from build123d import *

# Parameters (mm, degrees)
CROQUIS1_R              = 4.25
CROQUIS1_R_2            = 2
SALIENTE_EXTRUIR1_DEPTH = 14.2
CROQUIS2_W              = 12
CROQUIS2_H              = 162.31128511
CORTAR_EXTRUIR1_DEPTH   = 4
CROQUIS3_R              = 6.5
CORTAR_EXTRUIR2_DEPTH   = 8


with BuildPart() as part:
    # Croquis1 → Saliente-Extruir1 (new body)
    with BuildSketch(Plane.XY):
        with BuildLine():
            Line((69, -75), (56, -75))
            Line((56, -75), (56, -63))
            ThreePointArc((56, -63), (50, -57), (44, -63))
            Line((44, -63), (44, -75))
            Line((44, -75), (-44, -75))
            Line((-44, -75), (-44, -63))
            ThreePointArc((-44, -63), (-50, -57), (-56, -63))
            Line((-56, -63), (-56, -75))
            Line((-56, -75), (-69, -75))
            Line((-69, -75), (-69, 75))
            Line((-69, 75), (-56, 75))
            Line((-56, 75), (-56, 63))
            ThreePointArc((-56, 63), (-50, 57), (-44, 63))
            Line((-44, 63), (-44, 75))
            Line((-44, 75), (44, 75))
            Line((44, 75), (44, 63))
            ThreePointArc((44, 63), (50, 57), (56, 63))
            Line((56, 63), (56, 75))
            Line((56, 75), (69, 75))
            Line((69, 75), (69, -75))
        make_face()
        with Locations((-32.5, 40)):
            Circle(CROQUIS1_R, mode=Mode.SUBTRACT)
        with Locations((-32.5, 0)):
            Circle(CROQUIS1_R, mode=Mode.SUBTRACT)
        with Locations((-32.5, -40)):
            Circle(CROQUIS1_R, mode=Mode.SUBTRACT)
        with Locations((32.5, 40)):
            Circle(CROQUIS1_R, mode=Mode.SUBTRACT)
        with Locations((32.5, 0)):
            Circle(CROQUIS1_R, mode=Mode.SUBTRACT)
        with Locations((32.5, -40)):
            Circle(CROQUIS1_R, mode=Mode.SUBTRACT)
        with Locations((0, 65)):
            Circle(CROQUIS1_R_2, mode=Mode.SUBTRACT)
        Circle(CROQUIS1_R_2, mode=Mode.SUBTRACT)
        with Locations((0, -65)):
            Circle(CROQUIS1_R_2, mode=Mode.SUBTRACT)
    extrude(amount=SALIENTE_EXTRUIR1_DEPTH)

    # Croquis2 → Cortar-Extruir1 (cut)
    with BuildSketch(Plane.XY.offset(14.2)):
        with Locations((0, -0.838384737)):
            Rectangle(CROQUIS2_W, CROQUIS2_H)
    extrude(amount=-CORTAR_EXTRUIR1_DEPTH, mode=Mode.SUBTRACT)

    # Croquis3 → Cortar-Extruir2 (cut)
    with BuildSketch(Plane.XY.offset(14.2)):
        with Locations((-32.5, 40)):
            Circle(CROQUIS3_R)
        with Locations((-32.5, 0)):
            Circle(CROQUIS3_R)
        with Locations((-32.5, -40)):
            Circle(CROQUIS3_R)
        with Locations((32.5, 40)):
            Circle(CROQUIS3_R)
        with Locations((32.5, 0)):
            Circle(CROQUIS3_R)
        with Locations((32.5, -40)):
            Circle(CROQUIS3_R)
    extrude(amount=-CORTAR_EXTRUIR2_DEPTH, mode=Mode.SUBTRACT)


solid = part.part
Part model, mm, in its own coordinate system. A direction names the side the tool comes from. Round coordinates to 2 decimals unless told otherwise and drop trailing zeros. Order: outer loops, then holes, each group sorted by start corner. A loop starts at its lowest first (then second) coordinate and runs counter-clockwise, first axis right, second up. Notation, with made-up numbers: (-20.5, 88) -> (-7.5, 88) arc R6 cw to (-7.5, 98) -> close; hole circle Ø1 at (81.25, -5). An arc over 180 degrees is marked (long way). Put each result on its own line as item: value.
Q1. Pull direction Y, two halves, no side cores. Call faces 5 (the face through (56, -69, 7)), 6 (the face through (1, -75, 7)), 7 (the face through (33.9, -4.2, 6.2)), 8 (the face through (-39, 0, 10)): pulls with the +Y half, pulls with the -Y half, needs draft (parallel to the pull), parting line crosses it, or undercut.
From the geometry:
face 5: needs draft
face 6: pulls with the -Y half
face 7: undercut
face 8: undercut
Q2. Band-saw the part on C-C (y = -40). Give the cut face in (x, z), and give its area (3 significant figures).
From the geometry:
outline: (-69, 0) -> (-36.75, 0) -> (-36.75, 6.2) -> (-39, 6.2) -> (-39, 14.2) -> (-69, 14.2) -> close; (-28.25, 0) -> (28.25, 0) -> (28.25, 6.2) -> (26, 6.2) -> (26, 14.2) -> (6, 14.2) -> (6, 10.2) -> (-6, 10.2) -> (-6, 14.2) -> (-26, 14.2) -> (-26, 6.2) -> (-28.25, 6.2) -> close; (36.75, 0) -> (69, 0) -> (69, 14.2) -> (39, 14.2) -> (39, 6.2) -> (36.75, 6.2) -> close
area: 1,600 mm2
Q3. Wall check: line 1 (Y direction, x = -32.5, z = 11.25); line 2 (X direction, y = 69.5, z = 12); line 3 (X direction, y = 0, z = 3.25). Give the ranges that are in metal, low to high. Write a range as [from, to].
From the geometry:
line 1: y = [-75, -46.5], [-33.5, -6.5], [6.5, 33.5], [46.5, 75]
line 2: x = [-69, -56], [-44, -6], [6, 44], [56, 69]
line 3: x = [-69, -36.75], [-28.25, -2], [2, 28.25], [36.75, 69]
Q4. Tool access for faces 1 (the face through (3, 1, 10.2)), 2 (the face through (56, 69, 7)), 3 (the face through (31.654, -33.555, 10.256)), 4 (the face through (44, -69, 7)): list every direction of +Z, -Z, +X, -X, +Y, -Y with a clear straight run to the whole face (end or side of a thin tool).
From the geometry:
face 1: +Z, +Y, -Y
face 2: +Z, -Z, +Y
face 3: +Z
face 4: +Z, -Z, -Y
Q5. Pin check, flat tips, straight feed: pin 1 Ø5 at (x, y) = (-13, 32.5) entering from -Z; pin 2 Ø11 at (x, y) = (-32.5, 0) entering from +Z; pin 3 Ø4 at (x, z) = (48, 8) entering from -Y. Stop position of each tip, or through.
From the geometry:
pin 1: stops at z = 0
pin 2: stops at z = 6.2
pin 3: stops at y = -58.53
Q6. Band-saw the part on D-D (z = 3). State how many separate pieces and enclosed holes the cut face has, and give its area (3 significant figures).
From the geometry:
separate pieces: 1
enclosed holes: 9
area: 19,500 mm2
Q7. Band-saw the part on B-B (x = 0). Give the cut face in (y, z), and give its area (3 significant figures).
From the geometry:
outline: (-75, 0) -> (-67, 0) -> (-67, 10.2) -> (-75, 10.2) -> close; (-63, 0) -> (-2, 0) -> (-2, 10.2) -> (-63, 10.2) -> close; (2, 0) -> (63, 0) -> (63, 10.2) -> (2, 10.2) -> close; (67, 0) -> (75, 0) -> (75, 10.2) -> (67, 10.2) -> close
area: 1,410 mm2
Q8. Band-saw the part on A-A (y = -65). Give the cut face in (x, z).
From the geometry:
outline: (-69, 0) -> (-56, 0) -> (-56, 14.2) -> (-69, 14.2) -> close; (-44, 0) -> (-2, 0) -> (-2, 10.2) -> (-6, 10.2) -> (-6, 14.2) -> (-44, 14.2) -> close; (2, 0) -> (44, 0) -> (44, 14.2) -> (6, 14.2) -> (6, 10.2) -> (2, 10.2) -> close; (56, 0) -> (69, 0) -> (69, 14.2) -> (56, 14.2) -> close
